Study the drawing (mm; zero at the part's minimum x, y, z) and answer. A direction names the side the tool comes from. Give positions to 0.01 mm unless a question says otherwise; leave off trailing zeros. Write each loop counter-clockwise with the first axis right and the second up, starting at its lowest first coordinate (ties: lowest second). Pieces come first, ordered by that corner, then holes. Notation, with made-up numbers: (69, 21.5) -> (101, 21.5) arc R22 ccw to (101, 28.5) -> close; hole circle Ø6 at (-5, 77). An arc over 180 degrees is marked (long way). Use CSV: the item, a comma, the result in double quotes. Start each with the question number.
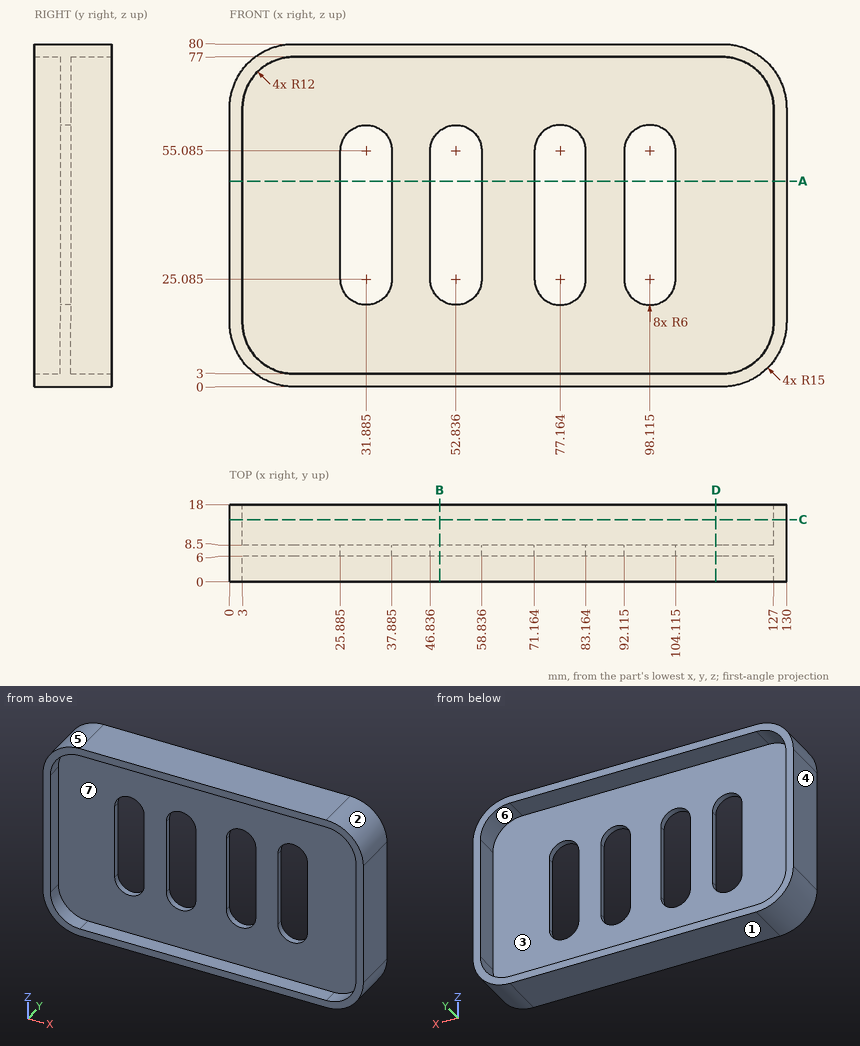
Q1. Straight lines are drawn through the part: L1, parallel to X at y = 7.75, z = 55 (1 decimal); L2, parallel to X at y = 7.75, z = 55.5; L3, parallel to Z at x = 59.5, y = 13.5. For each, find the intervals that lie inside material, in ascending order.
Q2. For the marked faces 5, 6 and 7, determine the directions among +Z, -Z, +X, -X, +Y, -Y from which every point of the face is accessible in a straight line to the end or side of a thin tool.
Q3. Section A-A on z = 48 is taken. Give the vertices of the cut face in (x, y) (1 decimal), then the cut area to 3 significant figures.
Q4. The mould has two halves that part along Z. Classify the marked faces 1, 2, 3 and 4: +Z half, -Z half, draft (parallel to the pull), parting line (faces both ways), or undercut.
Q5. Section B-B on x = 49 is taken. Give the vertices of the cut face in (y, z).
Q6. Section D-D on x = 113.5 is taken. Give the vertices of the cut face in (y, z).
Q7. Section C-C on y = 14.5 is taken. Give the vertices of the cut face in (x, z).
Output:
1,L1,"0 to 25.9, 37.9 to 46.8, 58.8 to 71.2, 83.2 to 92.1, 104.1 to 130"
1,L2,"0 to 25.9, 37.87 to 46.85, 58.82 to 71.18, 83.15 to 92.13, 104.1 to 130"
1,L3,"0 to 3, 77 to 80"
2,face 5,"+Z, -X, +Y, -Y"
2,face 6,"+Y"
2,face 7,"-Y"
3,outline,"(0, 0) -> (3, 0) -> (3, 6) -> (25.9, 6) -> (25.9, 8.5) -> (3, 8.5) -> (3, 18) -> (0, 18) -> close; (37.9, 6) -> (46.8, 6) -> (46.8, 8.5) -> (37.9, 8.5) -> close; (58.8, 6) -> (71.2, 6) -> (71.2, 8.5) -> (58.8, 8.5) -> close; (83.2, 6) -> (92.1, 6) -> (92.1, 8.5) -> (83.2, 8.5) -> close; (104.1, 6) -> (127, 6) -> (127, 0) -> (130, 0) -> (130, 18) -> (127, 18) -> (127, 8.5) -> (104.1, 8.5) -> close"
3,area,"298 mm²"
4,face 1,"-Z half"
4,face 2,"+Z half"
4,face 3,"undercut"
4,face 4,"draft"
5,outline,"(0, 0) -> (18, 0) -> (18, 3) -> (8.5, 3) -> (8.5, 20.47) -> (6, 20.47) -> (6, 3) -> (0, 3) -> close; (0, 77) -> (6, 77) -> (6, 59.7) -> (8.5, 59.7) -> (8.5, 77) -> (18, 77) -> (18, 80) -> (0, 80) -> close"
6,outline,"(0, 0) -> (18, 0) -> (18, 3) -> (8.5, 3) -> (8.5, 77) -> (18, 77) -> (18, 80) -> (0, 80) -> (0, 77) -> (6, 77) -> (6, 3) -> (0, 3) -> close"
7,outline,"(0, 15) arc R15 ccw to (15, 0) -> (115, 0) arc R15 ccw to (130, 15) -> (130, 65) arc R15 ccw to (115, 80) -> (15, 80) arc R15 ccw to (0, 65) -> close; hole (3, 15) arc R12 ccw to (15, 3) -> (115, 3) arc R12 ccw to (127, 15) -> (127, 65) arc R12 ccw to (115, 77) -> (15, 77) arc R12 ccw to (3, 65) -> close"
